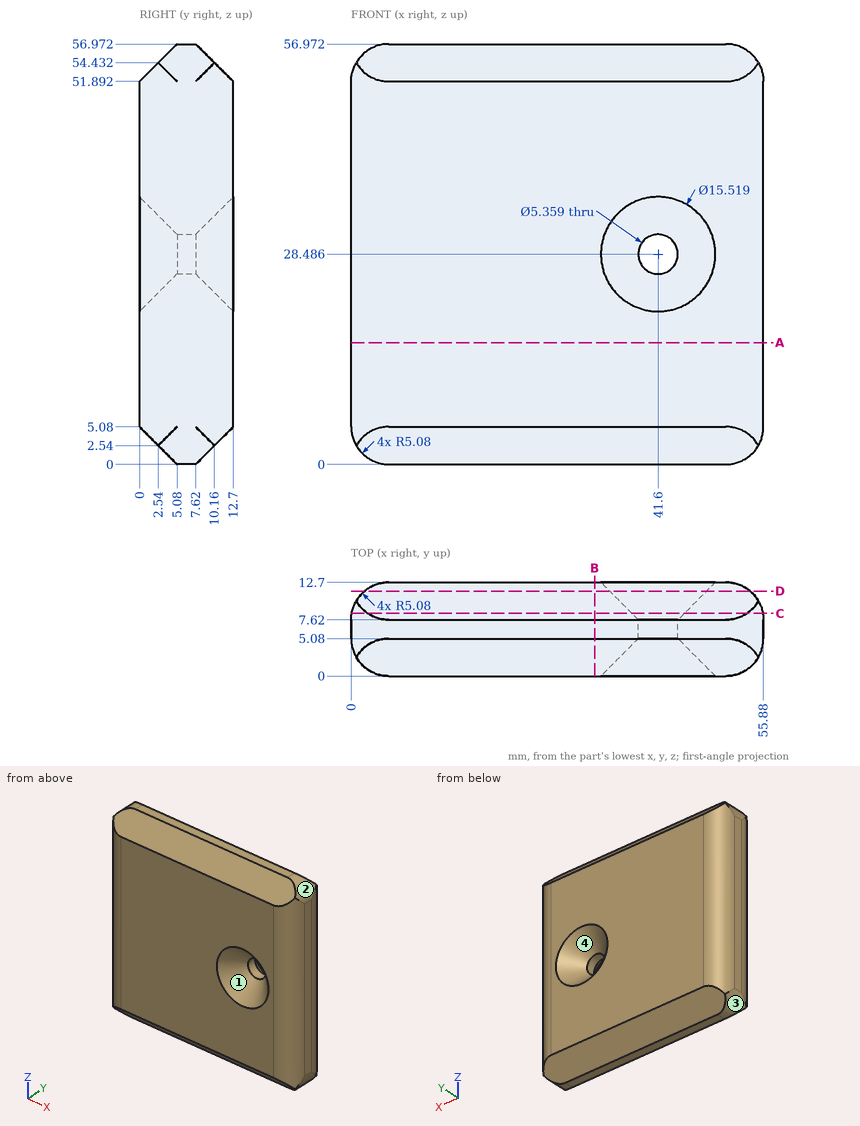
Source: three-view drawing plus pictorial views. Frame: mm from the lowest corner of the part. Round coordinates to 2 decimals unless told otherwise and drop trailing zeros. Loops run counter-clockwise (first coordinate to the right, second up) from the corner with the lowest first, then second, coordinate; pieces in that order, holes last.
Q1. Mould query, pull axis Z, two halves, no side actions, for the marked faces 1, 2, 3 and 4. Classes: pulls with the +Z half, pulls with the -Z half, needs draft (parallel to the pull), parting line crosses it, or undercut.
Q2. Ray query, line 1 (Z direction, x = 13, y = 3.25); line 2 (X direction, y = 7.5, z = 3) (1 decimal); line 3 (Z direction, x = 26, y = 8). Return the intervals inside material, ascending.
Q3. Section D-D, the plane y = 11.5. Return loops of the section in (x, z), plus the area to 3 significant figures.
Q4. First-contact query: P1, Ø2, axis at x = 43, y = 7, coming from the -Z side; P2, Ø3, axis at x = 41.6, z = 28.49, coming from the +Y side; P3, Ø2, axis at x = 22.5, y = 9.5, coming from the +Z side; P4, Ø1.5, axis at x = 42, y = 10, coming from the -Z side. Flat tips, straight axial feed; report the tip coordinate or a pass-through.
Q5. Section B-B, the plane x = 33. Return loops of the section in (y, z).
Q6. Section C-C, the plane y = 8.5. Return loops of the section in (x, z), plus the area to 3 significant figures.
Q7. Section A-A, the plane z = 16.5. Return loops of the section in (x, y).
Solutions:
1. face 1: undercut
1. face 2: pulls with the +Z half
1. face 3: pulls with the -Z half
1. face 4: undercut
2. line 1: z = 1.83 to 55.14
2. line 2: x = 0.4 to 55.4
2. line 3: z = 0.38 to 56.59
3. outline: (1.8, 3.88) - (54.08, 3.88) - (54.08, 53.09) - (1.8, 53.09) - close; hole circle Ø13.12 at (41.6, 28.49)
3. area: 2,440 mm2
4. P1: stops at z = 0
4. P2: passes through
4. P3: stops at z = 56.09
4. P4: stops at z = 1.63
5. outline: (0, 5.08) - (5.08, 0) - (7.62, 0) - (12.7, 5.08) - (12.7, 51.89) - (7.62, 56.97) - (5.08, 56.97) - (0, 51.89) - close
6. outline: (0.08, 4.2) arc R5.08 ccw to (2.22, 0.88) - (53.66, 0.88) arc R5.08 ccw to (55.8, 4.2) - (55.8, 52.77) arc R5.08 ccw to (53.66, 56.09) - (2.22, 56.09) arc R5.08 ccw to (0.08, 52.77) - close; hole circle Ø7.12 at (41.6, 28.49)
6. area: 3,030 mm2
7. outline: (0, 5.08) arc R5.08 ccw to (5.08, 0) - (50.8, 0) arc R5.08 ccw to (55.88, 5.08) - (55.88, 7.62) arc R5.08 ccw to (50.8, 12.7) - (5.08, 12.7) arc R5.08 ccw to (0, 7.62) - close
